For this review, use the dimensioned drawing (mm, ordinates from the lowest corner) and the shaded views. Coordinates: 2 decimals unless noted, no trailing zeros. Loops run counter-clockwise (first coordinate to the right, second up) from the corner with the lowest first, then second, coordinate; pieces in that order, holes last. Notation, with made-up numbers: M -13.75,2.25 L 41.25,2.25 A20 cw 41.25,25.25 Z; hole C -7,-36 d10. An arc over 180 degrees is marked long. One line per item, written item: value.
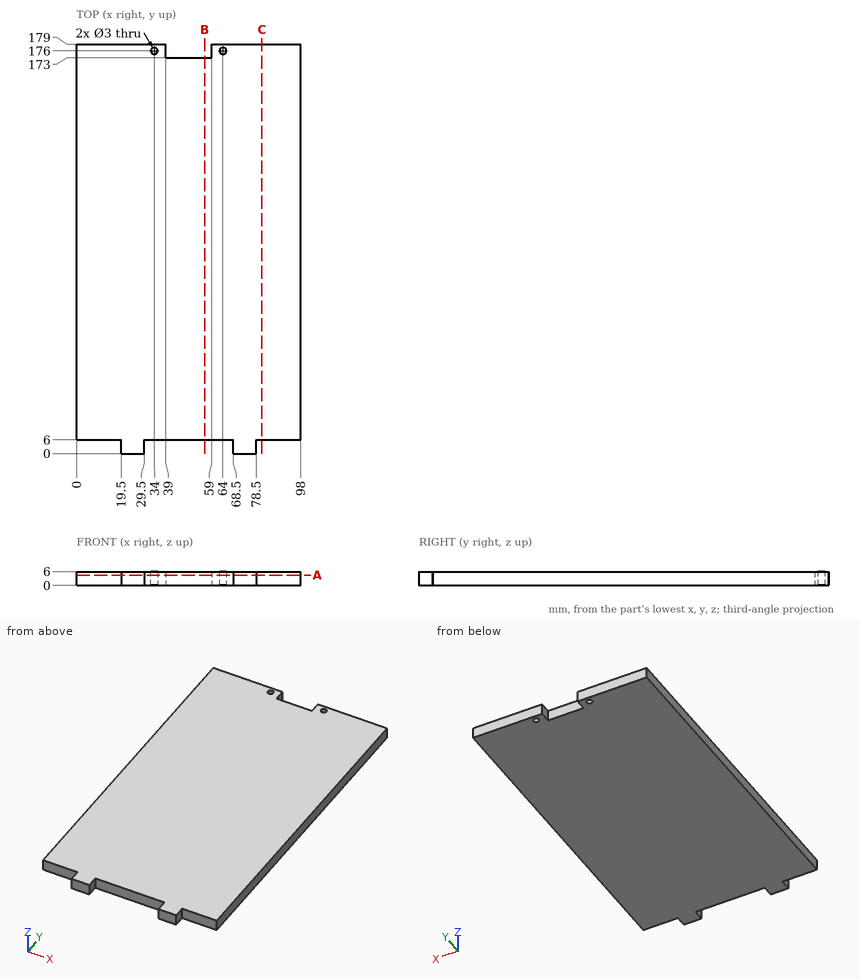
(1) Insertion check: pin 1 (1.8 mm diameter, centred on y = 4.5, z = 3, fed in from +X); pin 2 (1.8 mm diameter, centred on x = 64, y = 176, fed in from -Z); pin 3 (1.8 mm diameter, centred on x = 7.5, z = 4, fed in from -Y); pin 4 (3 mm diameter, centred on y = 3.5, z = 1.5, fed in from -X). Each pin has a flat end and moves straight along its axis. Give the tip position at first contact, or say it passes through.
Reply:
pin 1: stops at x = 78.5
pin 2: passes through
pin 3: stops at y = 6
pin 4: stops at x = 19.5
(2) To check wall thickness, follow line 1 along X through (y, z) = (176, 2.6); line 2 along Y through (x, z) = (64, 3.55); line 3 along Y through (x, z) = (32, 2). State the ranges of each line that lie inside material, in increasing order. Write a range as [from, to].
Reply:
line 1: x = [0, 32.5], [35.5, 39], [59, 62.5], [65.5, 98]
line 2: y = [6, 174.5], [177.5, 179]
line 3: y = [6, 179]
(3) We need section A-A on z = 4.55. State the section outline as (x, y) points.
Reply:
outline: M 0,6 L 19.5,6 L 19.5,0 L 29.5,0 L 29.5,6 L 68.5,6 L 68.5,0 L 78.5,0 L 78.5,6 L 98,6 L 98,179 L 59,179 L 59,173 L 39,173 L 39,179 L 0,179 Z; hole C 34,176 d3; hole C 64,176 d3
(4) We need section C-C on x = 81. State the section outline as (y, z) points.
Reply:
outline: M 6,0 L 179,0 L 179,6 L 6,6 Z
(5) We need section B-B on x = 56. State the section outline as (y, z) points.
Reply:
outline: M 6,0 L 173,0 L 173,6 L 6,6 Z
